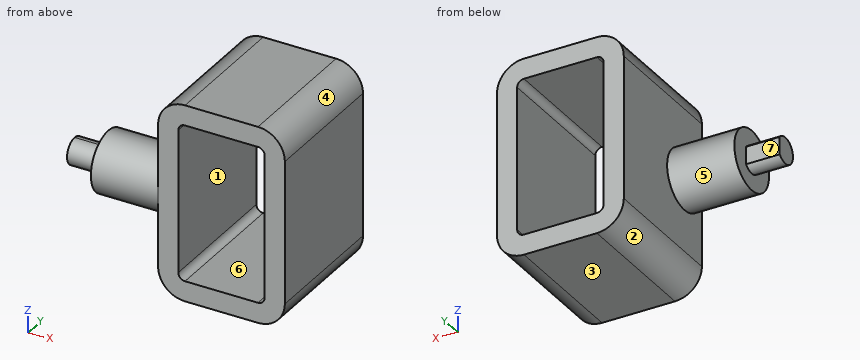
```python
from build123d import *

# Parameters (mm, degrees)
BOSS_EXTRUDE1_DEPTH = 20
SKETCH2_R           = 4.45
BOSS_EXTRUDE2_DEPTH = 10
BOSS_EXTRUDE3_DEPTH = 15


with BuildPart() as part:
    # Sketch1 → Boss-Extrude1 (new body)
    with BuildSketch(Plane(origin=(0, 0, 0), x_dir=(1, 0, 0), z_dir=(0, 1, 0))):
        with BuildLine():
            Line((-5.425, 14.625), (5.425, 14.625))
            ThreePointArc((5.425, 14.625), (8.253427125, 13.453427125), (9.425, 10.625))
            Line((9.425, 10.625), (9.425, -10.625))
            ThreePointArc((9.425, -10.625), (8.253427125, -13.453427125), (5.425, -14.625))
            Line((5.425, -14.625), (-5.425, -14.625))
            ThreePointArc((-5.425, -14.625), (-8.253427125, -13.453427125), (-9.425, -10.625))
            Line((-9.425, -10.625), (-9.425, 10.625))
            ThreePointArc((-9.425, 10.625), (-8.253427125, 13.453427125), (-5.425, 14.625))
        make_face()
        with BuildLine():
            Line((-5.425, 11.625), (5.425, 11.625))
            ThreePointArc((5.425, 11.625), (6.132106781, 11.332106781), (6.425, 10.625))
            Line((6.425, 10.625), (6.425, -10.625))
            ThreePointArc((6.425, -10.625), (6.132106781, -11.332106781), (5.425, -11.625))
            Line((5.425, -11.625), (-5.425, -11.625))
            ThreePointArc((-5.425, -11.625), (-6.132106781, -11.332106781), (-6.425, -10.625))
            Line((-6.425, -10.625), (-6.425, 10.625))
            ThreePointArc((-6.425, 10.625), (-6.132106781, 11.332106781), (-5.425, 11.625))
        make_face(mode=Mode.SUBTRACT)
    extrude(amount=BOSS_EXTRUDE1_DEPTH)

    # Sketch2 → Boss-Extrude2 (add)
    with BuildSketch(Plane.ZY.offset(9.425)):
        with Locations((0, 4.45)):
            Circle(SKETCH2_R)
        with BuildLine():
            Line((-1.303840481, 5.9), (1.303840481, 5.9))
            ThreePointArc((1.303840481, 5.9), (0, 2.5), (-1.303840481, 5.9))
        make_face(mode=Mode.SUBTRACT)
    extrude(amount=BOSS_EXTRUDE2_DEPTH)

    # Sketch2<4> → Boss-Extrude3 (add)
    with BuildSketch(Plane.ZY.offset(9.425)):
        with BuildLine():
            ThreePointArc((1.95, 4.45), (1.78114976, 5.243728878), (1.303840481, 5.9))
            Line((1.303840481, 5.9), (-1.303840481, 5.9))
            ThreePointArc((-1.303840481, 5.9), (-0.793728878, 2.66885024), (1.95, 4.45))
        make_face()
    extrude(amount=BOSS_EXTRUDE3_DEPTH)


solid = part.part
```
Model file for the job. Use its own axes, mm. Face numbers are marked on the shaded views. A direction names the side the tool comes from. Give positions to 0.01 mm unless a question says otherwise; leave off trailing zeros. Loops run counter-clockwise (first coordinate to the right, second up) from the corner with the lowest first, then second, coordinate; pieces in that order, holes last. Notation, with made-up numbers: (-23.5, 25.5) -> (9.5, 25.5) arc R18 ccw to (9.5, 53.5) -> close; hole circle Ø10 at (-31.5, 27.5). An arc over 180 degrees is marked (long way). Use CSV: the item, a comma, the result in double quotes. Start each with the question number.
1) Flat gauge pins, fed straight in: pin 1 Ø3 at (x, z) = (-21.5, 0.5) entering from +Y; pin 2 Ø1 at (x, z) = (-15.5, 1.5) entering from -Y; pin 3 Ø10 at (y, z) = (12.5, 1.5) entering from -X (3 decimals). Where does each tip first touch, or does it go through?
2) Slice it at B-B on x = 0.5. Give the cut face in (y, z) (3 decimals), plus the area to 3 significant figures.
3) Tool access for the marked faces 5, 6 and 7: list every direction of +Z, -Z, +X, -X, +Y, -Y with a clear straight run to the whole face (end or side of a thin tool).
4) Slice it at C-C on y = 16.5. Give the cut face in (x, z) (3 decimals), plus the area to 3 significant figures.
5) Wall check: line 1 (Z direction, x = 2.5, y = 2.5) (3 decimals); line 2 (X direction, y = 19.25, z = 8.25) (3 decimals); line 3 (Y direction, x = -19, z = -2.5). Give the ranges that are in metal, low to high.
6) Slice it at D-D on z = -3. Give the cut face in (x, y) (3 decimals), plus the area to 3 significant figures.
7) Mould opens along X. For the marked faces 1, 2, 3 and 4 say: released by +X, released by -X, zero draft, split by the parting line, or undercut.
8) Slice it at A-A on z = 5.5. Give the cut face in (x, y) (3 decimals).
Computed values:
1,pin 1,"stops at y = 5.9"
1,pin 2,"stops at y = 0.11"
1,pin 3,"stops at x = -19.425"
2,outline,"(0, -14.625) -> (20, -14.625) -> (20, -11.625) -> (0, -11.625) -> close; (0, 11.625) -> (20, 11.625) -> (20, 14.625) -> (0, 14.625) -> close"
2,area,"120 mm^2"
3,face 5,"-X"
3,face 6,"+Y, -Y"
3,face 7,"+Z, -Z, -X, +Y"
4,outline,"(-9.425, -10.625) arc R4 ccw to (-5.425, -14.625) -> (5.425, -14.625) arc R4 ccw to (9.425, -10.625) -> (9.425, 10.625) arc R4 ccw to (5.425, 14.625) -> (-5.425, 14.625) arc R4 ccw to (-9.425, 10.625) -> close; hole (-6.425, -10.625) arc R1 ccw to (-5.425, -11.625) -> (5.425, -11.625) arc R1 ccw to (6.425, -10.625) -> (6.425, 10.625) arc R1 ccw to (5.425, 11.625) -> (-5.425, 11.625) arc R1 ccw to (-6.425, 10.625) -> close"
4,area,"240 mm^2"
5,line 1,"z = -14.625 to -11.625, 11.625 to 14.625"
5,line 2,"x = -9.425 to -6.425, 6.425 to 9.425"
5,line 3,"y = 0.77 to 8.13"
6,outline,"(-19.425, 1.163) -> (-9.425, 1.163) -> (-9.425, 0) -> (-6.425, 0) -> (-6.425, 20) -> (-9.425, 20) -> (-9.425, 7.737) -> (-19.425, 7.737) -> close; (6.425, 0) -> (9.425, 0) -> (9.425, 20) -> (6.425, 20) -> close"
6,area,"186 mm^2"
7,face 1,"undercut"
7,face 2,"released by -X"
7,face 3,"zero draft"
7,face 4,"released by +X"
8,outline,"(-9.425, 0) -> (-6.425, 0) -> (-6.425, 20) -> (-9.425, 20) -> close; (6.425, 0) -> (9.425, 0) -> (9.425, 20) -> (6.425, 20) -> close"
